Verification items for the finished model (mm, model axes). Face numbers are marked on the shaded views. Coordinates: 2 decimals unless noted, no trailing zeros. Write each loop counter-clockwise with the first axis right and the second up, starting at its lowest first coordinate (ties: lowest second). Pieces come first, ordered by that corner, then holes. Notation, with made-up numbers: (10.5, 59) - (67.5, 59) arc R12 ccw to (67.5, 80) - close; hole circle Ø4 at (-33, -38). An arc over 180 degrees is marked (long way). Use CSV: the item, a comma, the result in double quotes. Start each with the question number.
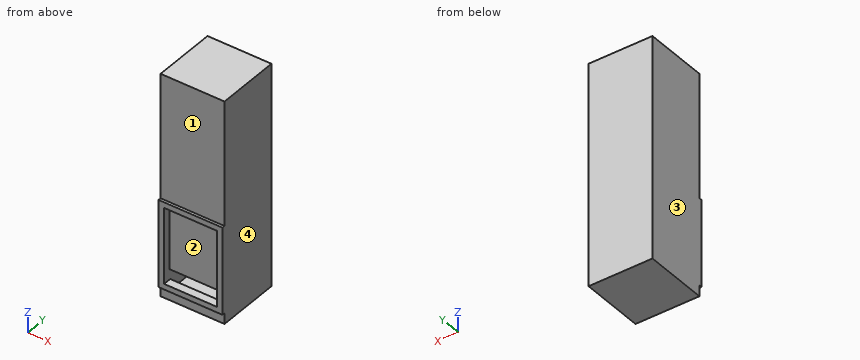
```python
from build123d import *

# Parameters (mm, degrees)
F0_W     = 584.2
F0_H     = 2032
F1_DEPTH = 584.2
F2_W     = 584.2
F2_H     = 796.1330711842
F3_DEPTH = 25.4
F4_T     = -50.8
F5_W     = 458.8919430971
F5_H     = 20.0611352921
F6_DEPTH = 581.66


with BuildPart() as f1:
    # F0 (on Front) → F1 (new body)
    with BuildSketch(Plane.XZ):
        with Locations((1.9479468465, 645.7104609217)):
            Rectangle(F0_W, F0_H)
    extrude(amount=F1_DEPTH)

    # F2 (on face) → F3 (join)
    with BuildSketch(Plane.XZ.offset(584.2)):
        with Locations((1.9479468465, 126.6288906336)):
            Rectangle(F2_W, F2_H)
    extrude(amount=F3_DEPTH)

    # F4
    f4_openings = [f1.faces().sort_by_distance(p)[0] for p in [
        (1.947947, -609.6, 126.628891),
    ]]
    offset(amount=F4_T, openings=f4_openings, kind=Kind.INTERSECTION)

    # F5 (on face) → F6 (join)
    with BuildSketch(Plane(origin=(0, 0, 473.8954262257), x_dir=(1, 0, 0), z_dir=(0, 0, -1))):
        with Locations((4.084430635, 551.7954230309)):
            Rectangle(F5_W, F5_H)
    extrude(amount=F6_DEPTH)


solid = f1.part
```
Q1. Gauge pin test, flat ends, axial feed: pin 1 (7.5 mm diameter, centred on x = -29.5, y = -596.5, fed in from -Z); pin 2 (7.5 mm diameter, centred on x = 1, y = -602, fed in from +Z). Record the tip position at first contact, or that the pin passes through.
Q2. Cross-section at D-D (x = -203). Record the cut outline in (y, z), plus the area to 3 significant figures.
Q3. Cross-section at B-B (z = 716). Record the cut outline in (x, y), plus the area to 3 significant figures.
Q4. Cross-section at A-A (z = 115). Record the cut outline in (x, y).
Q5. Cross-section at C-C (y = -318). Record the cut outline in (x, z).
Q6. Scan lines: line 1 along Z through (x, y) = (94, -436); line 2 along Y through (x, z) = (-212, 1280); line 3 along X through (y, z) = (-420.5, -111). Record each from-to range of solid material in increasing order. Write a range as from..to.
Q7. Release check for a two-part mould opening along X. For the marked faces 1, 2, 3 and 4 record: released by +X, released by -X, zero draft, split by the parting line, or undercut.
Reply:
1,pin 1,"z = -271.44"
1,pin 2,"z = 524.7"
2,outline,"(-609.6, -271.44) - (-584.2, -271.44) - (-584.2, -370.29) - (0, -370.29) - (0, 1661.71) - (-584.2, 1661.71) - (-584.2, 524.7) - (-609.6, 524.7) - (-609.6, 473.9) - (-561.83, 473.9) - (-561.83, -107.76) - (-541.76, -107.76) - (-541.76, 473.9) - (-533.4, 473.9) - (-533.4, 1610.91) - (-50.8, 1610.91) - (-50.8, -319.49) - (-533.4, -319.49) - (-533.4, -220.64) - (-609.6, -220.64) - close"
2,area,"234,000 mm^2"
3,outline,"(-290.15, -584.2) - (294.05, -584.2) - (294.05, 0) - (-290.15, 0) - close; hole (-239.35, -533.4) - (243.25, -533.4) - (243.25, -50.8) - (-239.35, -50.8) - close"
3,area,"108,000 mm^2"
4,outline,"(-290.15, -609.6) - (-239.35, -609.6) - (-239.35, -50.8) - (243.25, -50.8) - (243.25, -609.6) - (294.05, -609.6) - (294.05, 0) - (-290.15, 0) - close; (-225.36, -561.83) - (233.53, -561.83) - (233.53, -541.76) - (-225.36, -541.76) - close"
5,outline,"(-290.15, -370.29) - (294.05, -370.29) - (294.05, 1661.71) - (-290.15, 1661.71) - close; hole (-239.35, -319.49) - (243.25, -319.49) - (243.25, 1610.91) - (-239.35, 1610.91) - close"
6,line 1,"-370.29..-319.49, 1610.91..1661.71"
6,line 2,"-584.2..-533.4, -50.8..0"
6,line 3,"-290.15..-239.35, 243.25..294.05"
7,face 1,"zero draft"
7,face 2,"undercut"
7,face 3,"released by -X"
7,face 4,"released by +X"
